The model under review builds one solid part; all positions refer to its coordinate system, in mm. Coordinates: 2 decimals unless noted, no trailing zeros. Write each loop counter-clockwise with the first axis right and the second up, starting at its lowest first coordinate (ties: lowest second). Pieces come first, ordered by that corner, then holes.
```python
from build123d import *

# Parameters (mm, degrees)
ESQUISSE1_W             = 160
ESQUISSE1_H             = 100
ESQUISSE1_R             = 2.5
BOSS_EXTRU_1_DEPTH      = 10
ESQUISSE2_R             = 1.27
ENL_V_MAT_EXTRU_1_DEPTH = 189.944436277


with BuildPart() as part:
    # Esquisse1 → Boss.-Extru.1 (new body)
    with BuildSketch(Plane(origin=(0, 0, 0), x_dir=(1, 0, 0), z_dir=(0, 1, 0))):
        with Locations((80, 50)):
            Rectangle(ESQUISSE1_W, ESQUISSE1_H)
        with Locations(Location((5, 95, 0), (0, 0, 270))):
            Circle(ESQUISSE1_R, mode=Mode.SUBTRACT)
        with Locations(Location((5, 5, 0), (0, 0, 270))):
            Circle(ESQUISSE1_R, mode=Mode.SUBTRACT)
        with Locations(Location((155, 95, 0), (0, 0, 270))):
            Circle(ESQUISSE1_R, mode=Mode.SUBTRACT)
        with Locations(Location((155, 5, 0), (0, 0, 270))):
            Circle(ESQUISSE1_R, mode=Mode.SUBTRACT)
    extrude(amount=BOSS_EXTRU_1_DEPTH)

    # Esquisse2 → Enlèv. mat.-Extru.1 (cut, through all)
    with BuildSketch(Plane(origin=(0, 10, 0), x_dir=(1, 0, 0), z_dir=(0, 1, 0))):
        with Locations(Location((40.24, 74.13, 0), (0, 0, 270))):
            Circle(ESQUISSE2_R)
        with Locations(Location((38.97, 25.87, 0), (0, 0, 270))):
            Circle(ESQUISSE2_R)
        with Locations(Location((91.04, 30.95, 0), (0, 0, 270))):
            Circle(ESQUISSE2_R)
        with Locations(Location((121.92, 25.87, 0), (0, 0, 270))):
            Circle(ESQUISSE2_R)
        with Locations(Location((115.17, 74.13, 0), (0, 0, 270))):
            Circle(ESQUISSE2_R)
    extrude(amount=-ENL_V_MAT_EXTRU_1_DEPTH, mode=Mode.SUBTRACT)


solid = part.part
```
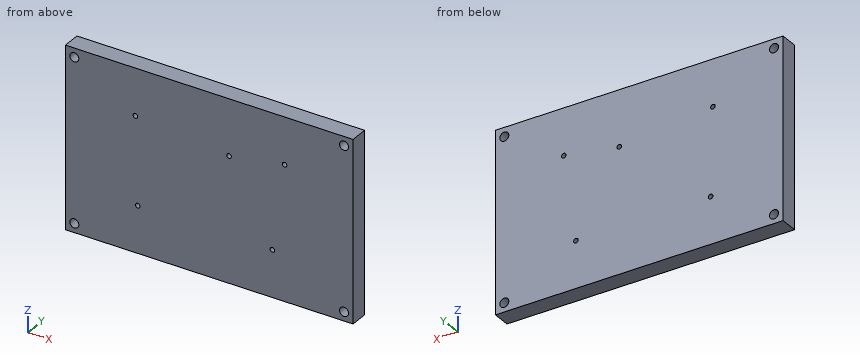
Item 1: Take a section at A-A, the plane x = 155. Write out the cut boundary in (y, z).
Solved:
outline: (0, -100) - (10, -100) - (10, -97.5) - (0, -97.5) - close; (0, -92.5) - (10, -92.5) - (10, -7.5) - (0, -7.5) - close; (0, -2.5) - (10, -2.5) - (10, 0) - (0, 0) - close
Item 2: For pin 1 (4 mm diameter, centred on x = 5, z = -95, fed in from +Y); pin 2 (1 mm diameter, centred on x = 20.5, z = -35.5, fed in from -Y), all flat-tipped, find the tip position at first contact; note any pin that passes through.
Solved:
pin 1: passes through
pin 2: stops at y = 0
Item 3: To check wall thickness, follow line 1 along X through (y, z) = (4.75, -74.13); line 2 along X through (y, z) = (7, -5); line 3 along Z through (x, y) = (115.17, 2.5). State the ranges of each line that lie inside material, in increasing order.
Solved:
line 1: x = 0 to 38.97, 41.51 to 113.9, 116.44 to 160
line 2: x = 0 to 2.5, 7.5 to 152.5, 157.5 to 160
line 3: z = -100 to -75.4, -72.86 to 0
